Could you check a few things on this model? Use its own coordinates, in mm. Give positions to 0.01 mm unless a question says otherwise; leave off trailing zeros. Loops run counter-clockwise (first coordinate to the right, second up) from the corner with the lowest first, then second, coordinate; pieces in that order, holes last.
1. Thinking about a two-plate mould opening in Y: for faces 1 (the cylindrical face through (75.547, 64.872, 1.014)), 2 (the flat face through (74.6, 98.4, 2)), which applies, +Y half, -Y half, draft (parallel to the pull), parting line (faces both ways), or undercut?
2. For P1, Ø18, axis at x = 77.5, y = 50, coming from the -Z side, with a flat end and sliding along its axis, tell me the tip position at first contact or that it passes through.
3. I need wall thicknesses on line 1 along Y through (x, z) = (77.5, 1.5); line 2 along X through (y, z) = (39, 1.35); line 3 along Y through (x, z) = (91, 1.25). Which ranges of each line are inside material? Lowest first, please.
4. Imagine slicing it at C-C (z = 0.5). List the corners of the cut face in (x, y) for me, plus the area to 3 significant figures.
```python
from build123d import *

# Parameters (mm, degrees)
ESQUISSE2_W             = 150
ESQUISSE2_H             = 100
BOSS_EXTRU_1_DEPTH      = 2
ESQUISSE3_W             = 146
ESQUISSE3_H             = 96
ENL_V_MAT_EXTRU_1_DEPTH = 0.0001
ESQUISSE4_R             = 15
ENL_V_MAT_EXTRU_2_DEPTH = 2.5


with BuildPart() as part:
    # Esquisse2 → Boss.-Extru.1 (new body)
    with BuildSketch(Plane.XY):
        with Locations((75, 50)):
            Rectangle(ESQUISSE2_W, ESQUISSE2_H)
    extrude(amount=BOSS_EXTRU_1_DEPTH)

    # Esquisse3 → Enlèv. mat.-Extru.1 (cut)
    with BuildSketch(Plane.XY.offset(2)):
        with Locations((75, 50)):
            Rectangle(ESQUISSE3_W, ESQUISSE3_H)
    extrude(amount=-ENL_V_MAT_EXTRU_1_DEPTH, mode=Mode.SUBTRACT)

    # Esquisse4 → Enlèv. mat.-Extru.2 (cut)
    with BuildSketch(Plane.XY.offset(1.9999)):
        with Locations((77.5, 50)):
            Circle(ESQUISSE4_R)
    extrude(amount=-ENL_V_MAT_EXTRU_2_DEPTH, mode=Mode.SUBTRACT)


solid = part.part
```
Derived:
1. face 1: undercut
1. face 2: draft
2. P1: passes through
3. line 1: y = 0 to 35, 65 to 100
3. line 2: x = 0 to 67.3, 87.7 to 150
3. line 3: y = 0 to 43.46, 56.54 to 100
4. outline: (0, 0) - (150, 0) - (150, 100) - (0, 100) - close; hole circle Ø30 at (77.5, 50)
4. area: 14,300 mm2
